from build123d import *

# Parameters (mm, degrees)
SKETCH1_R               = 2.75
BOSS_EXTRUDE1_DEPTH     = 14
SKETCH2_W               = 24
SKETCH2_H               = 32
CUT_EXTRUDE1_DEPTH      = 65
CUT_EXTRUDE1_DEPTH_BACK = 65
SKETCH3_W               = 64
SKETCH3_H               = 24
CUT_EXTRUDE2_DEPTH      = 22
SKETCH4_R               = 2.9
CUT_EXTRUDE3_DEPTH      = 2
CUT_EXTRUDE3_DEPTH_BACK = 2
SKETCH5_R               = 2.9
CUT_EXTRUDE4_DEPTH      = 2
CUT_EXTRUDE4_DEPTH_BACK = 2
SKETCH6_R               = 2.5
CUT_EXTRUDE5_DEPTH      = 14


with BuildPart() as part:
    # Sketch1 → Boss-Extrude1 (new body)
    with BuildSketch(Plane.XY):
        with BuildLine():
            Line((4.363786096, 0.902605737), (41.672757219, 17.026406116))
            ThreePointArc((41.672757219, 17.026406116), (42.63848659, 17.837594003), (43, 19.045884969))
            Line((43, 19.045884969), (43, 22))
            Line((43, 22), (0, 22))
            ThreePointArc((0, 22), (-4.209517756, 21.162674858), (-7.778174593, 18.778174593))
            Line((-7.778174593, 18.778174593), (-5.303300859, 16.303300859))
            ThreePointArc((-5.303300859, 16.303300859), (-6.652581249, 14.463114599), (-7.386058148, 12.302361333))
            Line((-7.386058148, 12.302361333), (-10.832885283, 12.910129954))
            ThreePointArc((-10.832885283, 12.910129954), (-6.819638592, 2.369094516), (4.363786096, 0.902605737))
        make_face()
        with Locations((0, 11)):
            Circle(SKETCH1_R, mode=Mode.SUBTRACT)
    extrude(amount=BOSS_EXTRUDE1_DEPTH)

    # Sketch2 → Cut-Extrude1 (cut, two sides)
    with BuildSketch(Plane(origin=(0, 0, 0), x_dir=(0, 0, -1), z_dir=(1, 0, 0))) as cut_extrude1_sk:
        with Locations((-7, 11)):
            Rectangle(SKETCH2_W, SKETCH2_H)
        with BuildLine():
            Line((-14, 20), (-3, 20))
            ThreePointArc((-3, 20), (-2.292893219, 19.707106781), (-2, 19))
            Line((-2, 19), (-2, 0))
            Line((-2, 0), (0, 0))
            Line((0, 0), (0, 20))
            ThreePointArc((0, 20), (-0.585786438, 21.414213562), (-2, 22))
            Line((-2, 22), (-14, 22))
            Line((-14, 22), (-14, 20))
        make_face(mode=Mode.SUBTRACT)
    extrude(amount=CUT_EXTRUDE1_DEPTH, mode=Mode.SUBTRACT)
    extrude(cut_extrude1_sk.sketch, amount=-CUT_EXTRUDE1_DEPTH_BACK, mode=Mode.SUBTRACT)

    # Sketch3 → Cut-Extrude2 (cut)
    with BuildSketch(Plane(origin=(0, 0, 0), x_dir=(-1, 0, 0), z_dir=(0, 1, 0))):
        with Locations((-16, 7)):
            Rectangle(SKETCH3_W, SKETCH3_H)
        with BuildLine():
            Line((11, 0), (11, 2))
            Line((11, 2), (-11, 2))
            Line((-11, 2), (-11, 10.5))
            ThreePointArc((-11, 10.5), (-12.025126266, 12.974873734), (-14.5, 14))
            Line((-14.5, 14), (-39.5, 14))
            ThreePointArc((-39.5, 14), (-41.974873734, 12.974873734), (-43, 10.5))
            Line((-43, 10.5), (-43, 0))
            Line((-43, 0), (11, 0))
        make_face(mode=Mode.SUBTRACT)
    extrude(amount=CUT_EXTRUDE2_DEPTH, mode=Mode.SUBTRACT)

    # Sketch4 → Cut-Extrude3 (cut, two sides)
    with BuildSketch(Plane(origin=(0, 22, 0), x_dir=(-1, 0, 0), z_dir=(0, 1, 0))) as cut_extrude3_sk:
        with Locations((-18, 8)):
            Circle(SKETCH4_R)
    extrude(amount=CUT_EXTRUDE3_DEPTH, mode=Mode.SUBTRACT)
    extrude(cut_extrude3_sk.sketch, amount=-CUT_EXTRUDE3_DEPTH_BACK, mode=Mode.SUBTRACT)

    # Sketch5 → Cut-Extrude4 (cut, two sides)
    with BuildSketch(Plane(origin=(0, 22, 0), x_dir=(-1, 0, 0), z_dir=(0, 1, 0))) as cut_extrude4_sk:
        with Locations((-36, 8)):
            Circle(SKETCH5_R)
    extrude(amount=CUT_EXTRUDE4_DEPTH, mode=Mode.SUBTRACT)
    extrude(cut_extrude4_sk.sketch, amount=-CUT_EXTRUDE4_DEPTH_BACK, mode=Mode.SUBTRACT)

    # Sketch6 → Cut-Extrude5 (cut)
    with BuildSketch(Plane.XY):
        with Locations((6, 22)):
            Circle(SKETCH6_R)
    extrude(amount=CUT_EXTRUDE5_DEPTH, mode=Mode.SUBTRACT)


solid = part.part
Design review of the part built by this model. Coordinates are the model's own, in mm. A direction names the side the tool comes from. Give positions to 0.01 mm unless a question says otherwise; leave off trailing zeros. Loops run counter-clockwise (first coordinate to the right, second up) from the corner with the lowest first, then second, coordinate; pieces in that order, holes last. Notation, with made-up numbers: (55.25, 62.25) -> (103.25, 62.25) arc R26 ccw to (103.25, 88.25) -> close; hole circle Ø6 at (18, -2). An arc over 180 degrees is marked (long way). One line per question, with ' | ' between items. Start each with the question number.
(1) We need section C-C (y = 11). State the section outline as (x, z) points, and give its area (3 significant figures).
(2) For faces 1 (the face through (-7, 18, 1)), 2 (the face through (22.757, 8.852, 0.986)), 3 (the face through (27, 20, 9)), list the 3-axis set-ups (+Z, -Z, +X, -X, +Y, -Y) from which the entire face can be reached by the end or side of a thin tool; tool diameter is ignored.
(3) For line 1 (Z direction, x = 24, y = 13.75); line 2 (Y direction, x = 15, z = 4); line 3 (Z direction, x = 18, y = 21), list the stretches that pass through material, from the lowest coordinate up.
(4) Insertion check: P1, Ø3.5, axis at x = 23.5, z = 6, coming from the -Y side; P2, Ø11, axis at x = 19.5, y = 10, coming from the +Z side; P3, Ø4.5, axis at x = 0, y = 11, coming from the +Z side; P4, Ø0.9, axis at y = 20, z = 5, coming from the -X side. Each pin has a flat end and moves straight along its axis. Give the tip position at first contact, or say it passes through.
(5) Draft analysis for pull direction Y (two halves, no side actions). For faces 4 (the face through (42.629, 17.823, 0.987)), 5 (the face through (-5, 20.8, 1.2)), 6 (the face through (33.234, 21.014, 8.871)), 7 (the face through (-6.64, 14.49, 0.99)), state which applies: +Y half, -Y half, draft (parallel to the pull), parting line (faces both ways), or undercut.
(6) We need section A-A (z = 8). State the section outline as (x, y) points, and give its area (3 significant figures).
(7) We need section D-D (x = 25.5). State the section outline as (y, z) points.
(8) We need section B-B (x = 20). State the section outline as (y, z) points, and give its area (3 significant figures).
The answers:
1) outline: (-11, 0) -> (-2.75, 0) -> (-2.75, 2) -> (-11, 2) -> close; (2.75, 0) -> (27.73, 0) -> (27.73, 2) -> (2.75, 2) -> close | area: 66.5 mm^2
2) face 1: +Z, -Z, -X | face 2: +Z, -Z, +X, -Y | face 3: +Z, +X, -X, -Y
3) line 1: z = 0 to 2 | line 2: y = 20 to 22 | line 3: z = 0.27 to 5.1, 10.9 to 14
4) P1: stops at y = 20 | P2: stops at z = 2 | P3: passes through | P4: stops at x = 11
5) face 4: -Y half | face 5: +Y half | face 6: draft | face 7: undercut
6) outline: (11, 20) -> (15.1, 20) -> (15.1, 22) -> (11, 22) -> close; (20.9, 20) -> (33.1, 20) -> (33.1, 22) -> (20.9, 22) -> close; (38.9, 20) -> (43, 20) -> (43, 22) -> (38.9, 22) -> close | area: 40.8 mm^2
7) outline: (10.04, 0) -> (20, 0) arc R2 ccw to (22, 2) -> (22, 14) -> (20, 14) -> (20, 3) arc R1 cw to (19, 2) -> (10.04, 2) -> close
8) outline: (7.66, 0) -> (20, 0) arc R2 ccw to (22, 2) -> (22, 5.9) -> (20, 5.9) -> (20, 3) arc R1 cw to (19, 2) -> (7.66, 2) -> close; (20, 10.1) -> (22, 10.1) -> (22, 14) -> (20, 14) -> close | area: 43.6 mm^2
